Build history of the part. All positions in model axes, mm. A direction names the side the tool comes from. Give positions to 0.01 mm unless a question says otherwise; leave off trailing zeros. Write each loop counter-clockwise with the first axis right and the second up, starting at its lowest first coordinate (ties: lowest second). Pieces come first, ordered by that corner, then holes. Notation, with made-up numbers: (1.5, 32.5) -> (58.5, 32.5) arc R14 ccw to (58.5, 39.5) -> close; hole circle Ø6 at (8, -4). An arc over 180 degrees is marked (long way). One line per question, with ' | ' between items. Start each with the question number.
(1) Drill centre lines: probe 1 along X at (y, z) = (11.5, 0); probe 2 along Y at (x, z) = (-17, 4.5); probe 3 along Z at (x, y) = (-1, 9.5). Where is each one in solid material? Low to high. Write a range as from..to.
(2) Pull direction X, two halves, no side cores. Call faces 4 (the cylindrical face through (10.81, 14.79, 34.34)), 5 (the flat face through (0, 0, 0)), 6 (the flat face through (0, -7, 11.725)): released by +X, released by -X, zero draft, split by the parting line, or undercut.
(3) Band-saw the part on A-A, the plane z = 0. Give the cut face in (x, y).
(4) Tool access for faces 1 (the flat face through (32.726, -12.4, 0.2)), 2 (the flat face through (-32.726, -12.4, 0.2)), 3 (the flat face through (0, -12.02, 0)): list every direction of +Z, -Z, +X, -X, +Y, -Y with a clear straight run to the whole face (end or side of a thin tool).
(5) Band-saw the part on C-C, the plane y = 9. Give the cut face in (x, z), and give its area (3 significant figures).
(6) Band-saw the part on B-B, the plane x = 0. Count the separate pieces of the cut face and the enclosed holes in it, and give its area (3 significant figures).
(7) Pin check, flat tips, straight feed: P1, Ø5, axis at y = 12.5, z = 4, coming from the -X side; P2, Ø1, axis at x = 23.5, y = 6, coming from the -Z side; P3, Ø5, axis at x = -5.5, y = -5.5, coming from the +Z side; P4, Ø2, axis at y = -9.5, z = 5.5, coming from the +X side. Stop position of each tip, or through.
from build123d import *

# Parameters (mm, degrees)
SKETCH_1_R          = 36
EXTRUDE_1_DEPTH     = 30
SKETCH_2_R          = 31
CUT_EXTRUDE_1_DEPTH = 30
FILLET_1_R          = 10
SKETCH_11_W         = 65.45159038682868
SKETCH_11_H         = 30
EXTRUDE_8_DEPTH     = 15
CUT_EXTRUDE_3_DEPTH = 84.18193869444944
CUT_EXTRUDE_4_DEPTH = 58.00000000000003
FILLET_2_SIZE       = 10


with BuildPart() as part:
    # 草圖1 → 填料-伸長1 (new body)
    with BuildSketch(Plane(origin=(0, 0, 0), x_dir=(1, 0, 0), z_dir=(0, 1, 0))):
        with Locations(Location((0, 0, 0), (0, 0, 270))):
            Circle(SKETCH_1_R)
    extrude(amount=EXTRUDE_1_DEPTH)

    # 草圖2 → 除料-伸長1 (cut)
    with BuildSketch(Plane(origin=(0, 30, 0), x_dir=(1, 0, 0), z_dir=(0, 1, 0))):
        with Locations(Location((0, 0, 0), (0, 0, 270))):
            Circle(SKETCH_2_R)
    extrude(amount=-CUT_EXTRUDE_1_DEPTH, mode=Mode.SUBTRACT)

    # 圓角1
    # the kernel refuses this fillet: 10 mm, written as the material it takes off along each edge
    with BuildSketch(Plane(origin=(0, 30, 0), x_dir=(-1.8e-16, 0, 1), z_dir=(-1, 0, -1.8e-16))) as fillet_1_piece_1:
        with BuildLine():
            CenterArc((41, -8.660254037844858), FILLET_1_R, 119.99999999999864, 60.000000000001364)
            Line((31.000000000000004, -8.660254037844858), (30.800000000000004, -8.660254037844858))
            Line((30.800000000000004, -8.660254037844858), (30.8, 0))
            Line((30.8, 0), (31, 0.1999999999999993))
            ThreePointArc((31, 0.1999999999999993), (33.5000000000001, 0.1999999999999993), (35.90000000000021, 0.17320508075653507))
            Line((35.90000000000021, 0.17320508075653507), (36.000000000000206, -3.5527e-13))
        make_face()
    revolve(axis=Axis((0, 30, 0), (0, 1, 0)), mode=Mode.SUBTRACT)

    # 草圖11 → 填料-伸長8 (add)
    with BuildSketch(Plane(origin=(0, 0, 0), x_dir=(1, 0, 0), z_dir=(0, 1, 0))):
        Rectangle(SKETCH_11_W, SKETCH_11_H)
    extrude(amount=-EXTRUDE_8_DEPTH)

    # 草圖16 → 除料-伸長3 (cut, through all)
    with BuildSketch(Plane.ZY.offset(32.72579519341434)):
        Polygon((-11.724999999999989, -2.02034535171655), (11.725000000000014, -2.02034535171655), (11.725000000000014, -12.02034535171655), (-11.724999999999985, -12.02034535171655), align=None)
    extrude(amount=-CUT_EXTRUDE_3_DEPTH, mode=Mode.SUBTRACT)

    # 草圖19 → 除料-伸長4 (cut)
    with BuildSketch(Plane.ZY.offset(32.72579519341434)):
        Polygon((-11.72500000000632, -6.624703450403075), (-12.725000000017417, -6.624703450403075), (-12.725000000017417, -5.624703450403075), (-13.725000000017417, -5.624703450403075), (-13.725000000017417, -8.624839762103937), (-12.725000000017417, -8.624839762103937), (-12.725000000017417, -7.624703450403074), (-11.72500000000632, -7.624703450403074), align=None)
    extrude(amount=-CUT_EXTRUDE_4_DEPTH, mode=Mode.SUBTRACT)

    # 圓角2
    # a fillet whose section is not a circle: 10 mm, written as the material it takes off along each edge
    with BuildSketch(Plane(origin=(52.129319932501346, 0, 15.000000000000002), x_dir=(0, -1, 0), z_dir=(-1, 0, 0))) as fillet_2_piece_1_section:
        with BuildLine():
            Bezier((FILLET_2_SIZE, 0), (0, 0), (0, -FILLET_2_SIZE), weights=[1, 2.3333333333333304, 1])
            Line((0, -FILLET_2_SIZE), (-FILLET_2_SIZE * 0.02, -FILLET_2_SIZE))
            Line((-FILLET_2_SIZE * 0.02, -FILLET_2_SIZE), (-FILLET_2_SIZE * 0.02, FILLET_2_SIZE * 0.02))
            Line((-FILLET_2_SIZE * 0.02, FILLET_2_SIZE * 0.02), (FILLET_2_SIZE, FILLET_2_SIZE * 0.02))
            Line((FILLET_2_SIZE, FILLET_2_SIZE * 0.02), (FILLET_2_SIZE, 0))
        make_face()
    fillet_2_piece_1 = extrude(amount=104.25863986500269, mode=Mode.PRIVATE)
    fillet_2_piece_1 = split(fillet_2_piece_1, bisect_by=Plane(origin=(52.129319932501346, 0, 15.000000000000002), z_dir=(0, -1, 0)), keep=Keep.TOP, mode=Mode.PRIVATE)
    fillet_2_piece_1 = fillet_2_piece_1 & Plane(origin=(0, 0, 0), x_dir=(-1.8e-16, 0, 1), z_dir=(0, 1, 0)) * Cylinder(31, 249, mode=Mode.PRIVATE)
    add(fillet_2_piece_1, mode=Mode.SUBTRACT)
    with BuildSketch(Plane(origin=(-52.12931993250088, 0, -14.999999999999998), x_dir=(0, -1, 0), z_dir=(1, 0, 0))) as fillet_2_piece_2_section:
        with BuildLine():
            Bezier((FILLET_2_SIZE, 0), (0, 0), (0, -FILLET_2_SIZE), weights=[1, 2.3333333333333304, 1])
            Line((0, -FILLET_2_SIZE), (-FILLET_2_SIZE * 0.02, -FILLET_2_SIZE))
            Line((-FILLET_2_SIZE * 0.02, -FILLET_2_SIZE), (-FILLET_2_SIZE * 0.02, FILLET_2_SIZE * 0.02))
            Line((-FILLET_2_SIZE * 0.02, FILLET_2_SIZE * 0.02), (FILLET_2_SIZE, FILLET_2_SIZE * 0.02))
            Line((FILLET_2_SIZE, FILLET_2_SIZE * 0.02), (FILLET_2_SIZE, 0))
        make_face()
    fillet_2_piece_2 = extrude(amount=104.25863986500174, mode=Mode.PRIVATE)
    fillet_2_piece_2 = split(fillet_2_piece_2, bisect_by=Plane(origin=(-52.12931993250088, 0, -14.999999999999998), z_dir=(0, -1, 0)), keep=Keep.TOP, mode=Mode.PRIVATE)
    fillet_2_piece_2 = fillet_2_piece_2 & Plane(origin=(0, 0, 0), x_dir=(-1.8e-16, 0, 1), z_dir=(0, 1, 0)) * Cylinder(31, 249, mode=Mode.PRIVATE)
    add(fillet_2_piece_2, mode=Mode.SUBTRACT)


solid = part.part
Results:
1) probe 1: x = -36..-31, 31..36 | probe 2: y = -15..-12.02, -2.02..0 | probe 3: z = -35.99..-30.98, 30.98..35.99
2) face 4: split by the parting line | face 5: undercut | face 6: zero draft
3) outline: (-36, 0) -> (-32.73, 0) -> (-32.73, -2.02) -> (32.73, -2.02) -> (32.73, 0) -> (36, 0) -> (36, 30) arc R10 ccw to (31, 21.34) -> (31, 0) -> (-31, 0) -> (-31, 21.34) arc R10 ccw to (-36, 30) -> close; (-32.73, -15) -> (32.73, -15) -> (32.73, -12.02) -> (-32.73, -12.02) -> close
4) face 1: +Z, -Z, +X, -Y | face 2: +Z, -Z, -X, -Y | face 3: +X, -X
5) outline: circle Ø72 at (0, 0); hole circle Ø62 at (0, 0) | area: 1,050 mm²
6) separate pieces: 3 | enclosed holes: 1 | area: 472 mm²
7) P1: stops at x = -35.97 | P2: stops at z = -27.69 | P3: stops at z = 14.98 | P4: passes through
